```python
from build123d import *

# Parameters (mm, degrees)
SKETCH1_R           = 2.38125
SKETCH1_W           = 3.2766
SKETCH1_H           = 3.2766
BOSS_EXTRUDE1_DEPTH = 4.7625


with BuildPart() as part:
    # Sketch1 → Boss-Extrude1 (new body)
    with BuildSketch(Plane.XY):
        with BuildLine():
            Line((0, 6.35), (63.5, 6.35))
            ThreePointArc((63.5, 6.35), (69.85, 0), (63.5, -6.35))
            Line((63.5, -6.35), (0, -6.35))
            ThreePointArc((0, -6.35), (-6.35, 0), (0, 6.35))
        make_face()
        with Locations(Location((0, 0, 0), (0, 0, 180))):
            Circle(SKETCH1_R, mode=Mode.SUBTRACT)
        with Locations(Location((20.32, 0, 0), (0, 0, 180))):
            Circle(SKETCH1_R, mode=Mode.SUBTRACT)
        with Locations((63.5, 0)):
            Rectangle(SKETCH1_W, SKETCH1_H, mode=Mode.SUBTRACT)
    extrude(amount=BOSS_EXTRUDE1_DEPTH)


solid = part.part
```
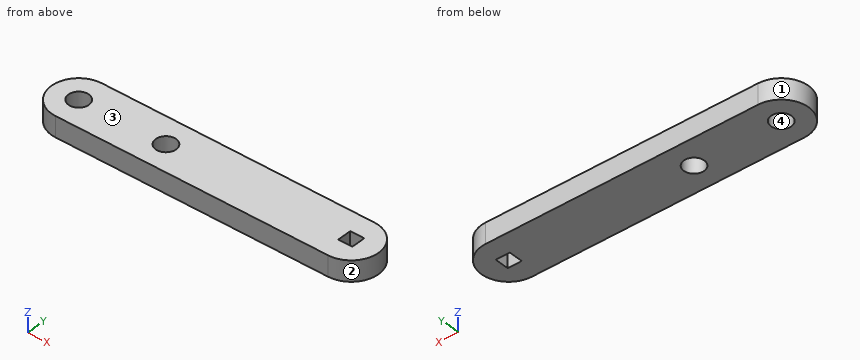
Model file for the job. Use its own axes, mm. Face numbers are marked on the shaded views. Give positions to 0.01 mm unless a question says otherwise; leave off trailing zeros. Loops run counter-clockwise (first coordinate to the right, second up) from the corner with the lowest first, then second, coordinate; pieces in that order, holes last. Notation, with made-up numbers: (67, 37.5) -> (123, 37.5) arc R26 ccw to (123, 65.5) -> close; hole circle Ø9 at (27.5, -5). An arc over 180 degrees is marked (long way). Write each question's results on one line, items separated by ' | '.
(1) Flat gauge pin, fed straight in: pin 1 Ø1.5 at (x, y) = (57, 3.5) entering from -Z. Where does the tip first touch, or does it go through?
Geometry results:
pin 1: stops at z = 0
(2) Pull direction X, two halves, no side cores. Call the marked faces 1, 2, 3 and 4: released by +X, released by -X, zero draft, split by the parting line, or undercut.
Geometry results:
face 1: released by -X | face 2: released by +X | face 3: zero draft | face 4: undercut
(3) Cut at D-D on y = 3.5. List the corners of the cut face in (x, z), and give its area (3 significant figures).
Geometry results:
outline: (-5.3, 0) -> (68.8, 0) -> (68.8, 4.76) -> (-5.3, 4.76) -> close | area: 353 mm²
(4) Cut at B-B on x = 20.32. List the corners of the cut face in (y, z), and give its area (3 significant figures).
Geometry results:
outline: (-6.35, 0) -> (-2.38, 0) -> (-2.38, 4.76) -> (-6.35, 4.76) -> close; (2.38, 0) -> (6.35, 0) -> (6.35, 4.76) -> (2.38, 4.76) -> close | area: 37.8 mm²
(5) Probe line 1 along Y through (x, z) = (20.32, 1.15); line 2 along X through (y, z) = (-4.25, 4.45). List the from-to ranges inside material, lowest first.
Geometry results:
line 1: y = -6.35 to -2.38, 2.38 to 6.35 | line 2: x = -4.72 to 68.22
(6) Cut at C-C on z = 1.35. List the corners of the cut face in (x, y).
Geometry results:
outline: (0, -6.35) -> (63.5, -6.35) arc R6.35 ccw to (63.5, 6.35) -> (0, 6.35) arc R6.35 ccw to start; hole circle Ø4.76 at (0, 0); hole circle Ø4.76 at (20.32, 0); hole (61.86, -1.64) -> (65.14, -1.64) -> (65.14, 1.64) -> (61.86, 1.64) -> close
(7) Cut at A-A on y = 0. List the corners of the cut face in (x, z), and give its area (3 significant figures).
Geometry results:
outline: (-6.35, 0) -> (-2.38, 0) -> (-2.38, 4.76) -> (-6.35, 4.76) -> close; (2.38, 0) -> (17.94, 0) -> (17.94, 4.76) -> (2.38, 4.76) -> close; (22.7, 0) -> (61.86, 0) -> (61.86, 4.76) -> (22.7, 4.76) -> close; (65.14, 0) -> (69.85, 0) -> (69.85, 4.76) -> (65.14, 4.76) -> close | area: 302 mm²
